```python
from build123d import *

# Parameters (mm, degrees)
EXTRUDE_1_DEPTH     = 6
SKETCH_3_R          = 1.4
CUT_EXTRUDE_1_DEPTH = 6
SKETCH_4_R          = 5
EXTRUDE_2_DEPTH     = 12
CUT_EXTRUDE_2_DEPTH = 12


with BuildPart() as part:
    # 草图2 → 凸台-拉伸1 (new body)
    with BuildSketch(Plane(origin=(0, 0, 0), x_dir=(1, 0, 0), z_dir=(0, 1, 0))):
        with BuildLine():
            Line((-1.1, 10.341663309), (-1.3, 12.432216214))
            ThreePointArc((-1.3, 12.432216214), (0, 12.5), (1.3, 12.432216214))
            Line((1.3, 12.432216214), (1.1, 10.341663309))
            ThreePointArc((1.1, 10.341663309), (2.691718069, 10.045628593), (4.21820371, 9.506143143))
            Line((4.21820371, 9.506143143), (5.090275082, 11.416615067))
            ThreePointArc((5.090275082, 11.416615067), (6.25, 10.825317547), (7.341941132, 10.116615067))
            Line((7.341941132, 10.116615067), (6.123459599, 8.406143143))
            ThreePointArc((6.123459599, 8.406143143), (7.353910524, 7.353910524), (8.406143143, 6.123459599))
            Line((8.406143143, 6.123459599), (10.116615067, 7.341941132))
            ThreePointArc((10.116615067, 7.341941132), (10.825317547, 6.25), (11.416615067, 5.090275082))
            Line((11.416615067, 5.090275082), (9.506143143, 4.21820371))
            ThreePointArc((9.506143143, 4.21820371), (10.045628593, 2.691718069), (10.341663309, 1.1))
            Line((10.341663309, 1.1), (12.432216214, 1.3))
            ThreePointArc((12.432216214, 1.3), (12.5, 0), (12.432216214, -1.3))
            Line((12.432216214, -1.3), (10.341663309, -1.1))
            ThreePointArc((10.341663309, -1.1), (10.045628593, -2.691718069), (9.506143143, -4.21820371))
            Line((9.506143143, -4.21820371), (11.416615067, -5.090275082))
            ThreePointArc((11.416615067, -5.090275082), (10.825317547, -6.25), (10.116615067, -7.341941132))
            Line((10.116615067, -7.341941132), (8.406143143, -6.123459599))
            ThreePointArc((8.406143143, -6.123459599), (7.353910524, -7.353910524), (6.123459599, -8.406143143))
            Line((6.123459599, -8.406143143), (7.341941132, -10.116615067))
            ThreePointArc((7.341941132, -10.116615067), (6.25, -10.825317547), (5.090275082, -11.416615067))
            Line((5.090275082, -11.416615067), (4.21820371, -9.506143143))
            ThreePointArc((4.21820371, -9.506143143), (2.691718069, -10.045628593), (1.1, -10.341663309))
            Line((1.1, -10.341663309), (1.3, -12.432216214))
            ThreePointArc((1.3, -12.432216214), (0, -12.5), (-1.3, -12.432216214))
            Line((-1.3, -12.432216214), (-1.1, -10.341663309))
            ThreePointArc((-1.1, -10.341663309), (-2.691718069, -10.045628593), (-4.21820371, -9.506143143))
            Line((-4.21820371, -9.506143143), (-5.090275082, -11.416615067))
            ThreePointArc((-5.090275082, -11.416615067), (-6.25, -10.825317547), (-7.341941132, -10.116615067))
            Line((-7.341941132, -10.116615067), (-6.123459599, -8.406143143))
            ThreePointArc((-6.123459599, -8.406143143), (-7.353910524, -7.353910524), (-8.406143143, -6.123459599))
            Line((-8.406143143, -6.123459599), (-10.116615067, -7.341941132))
            ThreePointArc((-10.116615067, -7.341941132), (-10.825317547, -6.25), (-11.416615067, -5.090275082))
            Line((-11.416615067, -5.090275082), (-9.506143143, -4.21820371))
            ThreePointArc((-9.506143143, -4.21820371), (-10.045628593, -2.691718069), (-10.341663309, -1.1))
            Line((-10.341663309, -1.1), (-12.432216214, -1.3))
            ThreePointArc((-12.432216214, -1.3), (-12.5, 0), (-12.432216214, 1.3))
            Line((-12.432216214, 1.3), (-10.341663309, 1.1))
            ThreePointArc((-10.341663309, 1.1), (-10.045628593, 2.691718069), (-9.506143143, 4.21820371))
            Line((-9.506143143, 4.21820371), (-11.416615067, 5.090275082))
            ThreePointArc((-11.416615067, 5.090275082), (-10.825317547, 6.25), (-10.116615067, 7.341941132))
            Line((-10.116615067, 7.341941132), (-8.406143143, 6.123459599))
            ThreePointArc((-8.406143143, 6.123459599), (-7.353910524, 7.353910524), (-6.123459599, 8.406143143))
            Line((-6.123459599, 8.406143143), (-7.341941132, 10.116615067))
            ThreePointArc((-7.341941132, 10.116615067), (-6.25, 10.825317547), (-5.090275082, 11.416615067))
            Line((-5.090275082, 11.416615067), (-4.21820371, 9.506143143))
            ThreePointArc((-4.21820371, 9.506143143), (-2.691718069, 10.045628593), (-1.1, 10.341663309))
        make_face()
    extrude(amount=EXTRUDE_1_DEPTH)

    # 草图3 → 切除-拉伸1 (cut)
    with BuildSketch(Plane(origin=(0, 6, 0), x_dir=(1, 0, 0), z_dir=(0, 1, 0))):
        with Locations(Location((0, 0, 0), (0, 0, 270))):
            Circle(SKETCH_3_R)
    extrude(amount=-CUT_EXTRUDE_1_DEPTH, mode=Mode.SUBTRACT)

    # 草图4 → 凸台-拉伸2 (add)
    with BuildSketch(Plane(origin=(0, 6, 0), x_dir=(1, 0, 0), z_dir=(0, 1, 0))):
        with Locations(Location((0, 0, 0), (0, 0, 270))):
            Circle(SKETCH_4_R)
    extrude(amount=EXTRUDE_2_DEPTH)

    # 草图5 → 切除-拉伸2 (cut)
    with BuildSketch(Plane(origin=(0, 18, 0), x_dir=(1, 0, 0), z_dir=(0, 1, 0))):
        with BuildLine():
            Line((-1, -1.118033989), (1, -1.118033989))
            ThreePointArc((1, -1.118033989), (0, 1.5), (-1, -1.118033989))
        make_face()
    extrude(amount=-CUT_EXTRUDE_2_DEPTH, mode=Mode.SUBTRACT)

    # 草图7 → 旋转1 (revolve)
    with BuildSketch(Plane(origin=(0, 0, 0), x_dir=(0, 0, -1), z_dir=(1, 0, 0)), mode=Mode.PRIVATE) as revolve_1_sk:
        with BuildLine():
            Line((5, 9), (12.432216214, 9))
            Line((12.432216214, 9), (12.432216214, 8.511911797))
            ThreePointArc((12.432216214, 8.511911797), (11.390525649, 7.5), (12.432216214, 6.488088203))
            Line((12.432216214, 6.488088203), (12.432216214, 6))
            Line((12.432216214, 6), (5, 6))
            Line((5, 6), (5, 9))
        make_face()
    revolve(revolve_1_sk.sketch.rotate(Axis((0, 19.919763073, 0), (0, -1, 0)), 180), axis=Axis((0, 19.919763073, 0), (0, -1, 0)))


solid = part.part
```
Geometry: final body of the model. Coordinates: model frame, mm. A direction names the side the tool comes from. Round coordinates to 2 decimals unless told otherwise and drop trailing zeros. Order: outer loops, then holes, each group sorted by start corner. A loop starts at its lowest first (then second) coordinate and runs counter-clockwise, first axis right, second up. Notation, with made-up numbers: (19.5, -12) - (44.5, -12) arc R20 cw to (44.5, 15) - close; hole circle Ø4 at (60.5, -7.5). An arc over 180 degrees is marked (long way). Use CSV: the item, a comma, the result in double quotes. Start each with the question number.
Q1. Material intervals for line 1 along Z through (x, y) = (0, 11.25); line 2 along Z through (x, y) = (0, 2.8); line 3 along X through (y, z) = (11.75, 0), sorted ascending. Write a range as from..to.
Q2. Access query for faces 5 (the face through (4.66, 2.96, 10.47)), 6 (the face through (-8, 6, -8)), 7 (the face through (-6.724, 2.958, -9.249)), 8 (the face through (10.47, 2.96, -4.66)). Directions: +Z, -Z, +X, -X, +Y, -Y. A direction counts if a zero-diameter tool reaches every point of the face in a straight line with its end or side. Return the directions, or none.
Q3. Section query B-B (x = 0). Return loops of the section in (y, z), and give its area (3 significant figures).
Q4. Section query A-A (z = 0). Return loops of the section in (x, y), and give its area (3 significant figures).
Q5. Mould query, pull axis Z, two halves, no side actions, for faces 1 (the face through (-10.04, 2.96, 2.71)), 2 (the face through (-12.5, 3, 0)), 3 (the face through (10.45, 2.96, 4.65)), 4 (the face through (1.2, 18, -1.2)). Classes: +Z half, -Z half, draft (parallel to the pull), parting line (faces both ways), or undercut.
Q6. First-contact query: pin 1 (1.4 mm diameter, centred on x = -11, z = -3.5, fed in from -Y); pin 2 (1.1 mm diameter, centred on x = 6.5, z = -11, fed in from +Y); pin 3 (1.6 mm diameter, centred on x = 0, y = 14, fed in from -Z). Flat tips, straight axial feed; report the tip coordinate or a pass-through.
Q7. Section query C-C (y = 14.25). Return loops of the section in (x, z).
Result set:
1,line 1,"z = -5..-1.5, 1.12..5"
1,line 2,"z = -12.5..-1.4, 1.4..12.5"
1,line 3,"x = -5..-1.5, 1.5..5"
2,face 5,"+Z, -Y"
2,face 6,"-Y"
2,face 7,"-X, -Y"
2,face 8,"+X, -Y"
3,outline,"(0, -12.5) - (6, -12.5) - (6, -12.43) - (6.49, -12.43) arc R1.01 cw (long way) to (8.51, -12.43) - (9, -12.43) - (9, -5) - (18, -5) - (18, -1.5) - (6, -1.5) - (6, -1.4) - (0, -1.4) - close; (0, 1.4) - (6, 1.4) - (6, 1.12) - (18, 1.12) - (18, 5) - (9, 5) - (9, 12.43) - (8.51, 12.43) arc R1.01 cw (long way) to (6.49, 12.43) - (6, 12.43) - (6, 12.5) - (0, 12.5) - close"
3,area,"263 mm2"
4,outline,"(-12.5, 0) - (-1.4, 0) - (-1.4, 6) - (-1.5, 6) - (-1.5, 18) - (-5, 18) - (-5, 9) - (-12.43, 9) - (-12.43, 8.51) arc R1.01 cw (long way) to (-12.43, 6.49) - (-12.43, 6) - (-12.5, 6) - close; (1.4, 0) - (12.5, 0) - (12.5, 6) - (12.43, 6) - (12.43, 6.49) arc R1.01 cw (long way) to (12.43, 8.51) - (12.43, 9) - (5, 9) - (5, 18) - (1.5, 18) - (1.5, 6) - (1.4, 6) - close"
4,area,"258 mm2"
5,face 1,"undercut"
5,face 2,"parting line"
5,face 3,"undercut"
5,face 4,"draft"
6,pin 1,"stops at y = 6"
6,pin 2,"stops at y = 9"
6,pin 3,"stops at z = -5"
7,outline,"circle Ø10 at (0, 0); hole (-1, 1.12) arc R1.5 ccw (long way) to (1, 1.12) - close"
